Here's how the part is built. I have some questions about the finished solid (model axes, mm). Face numbers are marked on the shaded views. Round coordinates to 2 decimals unless told otherwise and drop trailing zeros. Loops run counter-clockwise (first coordinate to the right, second up) from the corner with the lowest first, then second, coordinate; pieces in that order, holes last. Notation, with made-up numbers: M -39.75,49.5 L -5.75,49.5 A22 cw -5.75,73.5 Z; hole C 4,36.5 d4. An arc over 180 degrees is marked long. Answer as a JSON object with one key per item and string values.
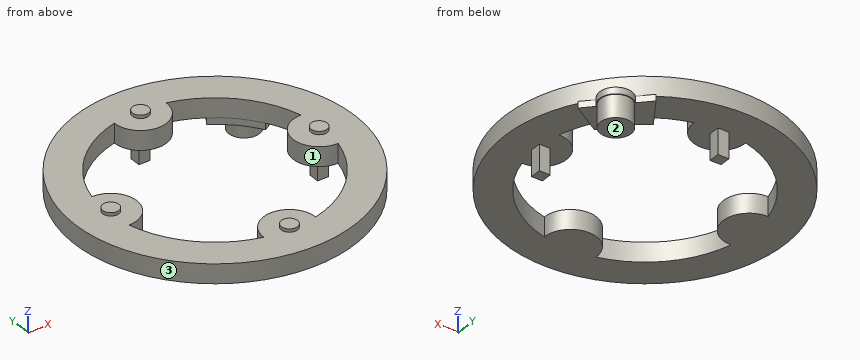
from build123d import *

# Parameters (mm, degrees)
SKETCH1_R           = 110.363
BOSS_EXTRUDE1_DEPTH = 15.24
SKETCH2_R           = 6.35
BOSS_EXTRUDE2_DEPTH = 2.54
SKETCH3_W           = 8.636
SKETCH3_H           = 8.636
BOSS_EXTRUDE3_DEPTH = 20.32
SKETCH4_W           = 8.7122
SKETCH4_H           = 8.636
BOSS_EXTRUDE4_DEPTH = 20.32
BOSS_EXTRUDE5_START = 5.08
BOSS_EXTRUDE5_DEPTH = 5.08
BOSS_EXTRUDE6_DEPTH = 5.08
SKETCH7_R           = 12.070643518
BOSS_EXTRUDE7_DEPTH = 17.78
SCALE2_SCALE        = 1.5


with BuildPart() as part:
    # Sketch1 → Boss-Extrude1 (new body)
    with BuildSketch(Plane.XY):
        Circle(SKETCH1_R)
        with BuildLine():
            ThreePointArc((-20.468919413, 82.460503922), (-60.07791345, 60.07791345), (-82.460503922, 20.468919413))
            ThreePointArc((-82.460503922, 20.468919413), (-61.684540449, 0), (-82.460503922, -20.468919413))
            ThreePointArc((-82.460503922, -20.468919413), (-60.07791345, -60.07791345), (-20.468919413, -82.460503922))
            ThreePointArc((-20.468919413, -82.460503922), (0, -61.684540449), (20.468919413, -82.460503922))
            ThreePointArc((20.468919413, -82.460503922), (60.07791345, -60.07791345), (82.460503922, -20.468919413))
            ThreePointArc((82.460503922, -20.468919413), (61.684540449, 0), (82.460503922, 20.468919413))
            ThreePointArc((82.460503922, 20.468919413), (60.07791345, 60.07791345), (20.468919413, 82.460503922))
            ThreePointArc((20.468919413, 82.460503922), (0, 61.684540449), (-20.468919413, 82.460503922))
        make_face(mode=Mode.SUBTRACT)
    extrude(amount=BOSS_EXTRUDE1_DEPTH)

    # Sketch2 → Boss-Extrude2 (add)
    with BuildSketch(Plane.XY.offset(15.24)):
        with Locations((0, 82.155728736)):
            Circle(SKETCH2_R)
        with Locations((82.155728736, 0)):
            Circle(SKETCH2_R)
        with Locations((0, -82.155728736)):
            Circle(SKETCH2_R)
        with Locations((-82.155728736, 0)):
            Circle(SKETCH2_R)
    extrude(amount=BOSS_EXTRUDE2_DEPTH)

    # Sketch3 → Boss-Extrude3 (add)
    with BuildSketch(Plane(origin=(0, 0, 0), x_dir=(-1, 0, 0), z_dir=(0, 0, -1))):
        with Locations((-82.155728736, 0)):
            Rectangle(SKETCH3_W, SKETCH3_H)
    extrude(amount=BOSS_EXTRUDE3_DEPTH)

    # Sketch4 → Boss-Extrude4 (add)
    with BuildSketch(Plane(origin=(0, 0, 0), x_dir=(-1, 0, 0), z_dir=(0, 0, -1))):
        with Locations((0, 82.155728736)):
            Rectangle(SKETCH4_W, SKETCH4_H)
    extrude(amount=BOSS_EXTRUDE4_DEPTH)

    # Sketch5 → Boss-Extrude5 (add)
    with BuildSketch(Plane(origin=(0, 0, 0), x_dir=(-1, 0, 0), z_dir=(0, 0, -1)).offset(BOSS_EXTRUDE5_START)):
        with BuildLine():
            Line((-72.079043308, 44.981361527), (-95.54887759, 59.627853106))
            Line((-95.54887759, 59.627853106), (-59.627853106, 95.54887759))
            Line((-59.627853106, 95.54887759), (-44.981361527, 72.079043308))
            ThreePointArc((-44.981361527, 72.079043308), (-60.07791345, 60.07791345), (-72.079043308, 44.981361527))
        make_face()
    extrude(amount=-BOSS_EXTRUDE5_DEPTH)

    # Sketch6 → Boss-Extrude6 (add)
    with BuildSketch(Plane(origin=(0, 0, -5.08), x_dir=(-1, 0, 0), z_dir=(0, 0, -1))):
        with BuildLine():
            Line((-87.073217452, 68.103513244), (-69.11270521, 86.064025486))
            ThreePointArc((-69.11270521, 86.064025486), (-87.073217452, 86.064025486), (-87.073217452, 68.103513244))
        make_face()
    extrude(amount=-BOSS_EXTRUDE6_DEPTH)

    # Sketch7 → Boss-Extrude7 (add)
    with BuildSketch(Plane(origin=(0, 0, -5.08), x_dir=(-1, 0, 0), z_dir=(0, 0, -1))):
        with Locations(Location((-78.092961331, 77.083769365, 0), (0, 0, 180))):
            Circle(SKETCH7_R)
    extrude(amount=BOSS_EXTRUDE7_DEPTH)


with BuildPart() as part_1:
    # Scale2: scaled about (4.191580163, 4.163736675, 6.658412252)
    add(part.part.scale(SCALE2_SCALE).moved(Location((-2.095790082, -2.081868337, -3.329206126))))


solid = part_1.part
Item 1: I'm going to push flat-ended pins straight in: pin 1 Ø10.5 at (x, z) = (-2.5, -18) entering from -Y; pin 2 Ø4 at (y, z) = (120, -13) entering from -X; pin 3 Ø14.5 at (x, z) = (-4.5, -25) entering from +Y. Where does each tip first touch, or does it pass through?
Resolved:
{"pin 1": "y = 114.67", "pin 2": "x = -8.63", "pin 3": "y = 127.63"}
Item 2: Please list where these lines run through material, in increasing order: probe 1 along X at (y, z) = (-6, -32); probe 2 along X at (y, z) = (-13.5, -3); probe 3 along Z at (x, y) = (-147.5, 6). Write a range as from..to.
Resolved:
{"probe 1": "114.66..127.61", "probe 2": "-167.25..-96.82, 92.63..163.05", "probe 3": "-3.33..19.53"}
Item 3: I want a section at C-C, the plane z = -27.5. Please give me the cut outline in (x, y), then the cut area to 3 significant figures.
Resolved:
{"outline": "M -8.63,114.67 L 4.44,114.67 L 4.44,127.63 L -8.63,127.63 Z; C 115.04,113.54 d36.21; M 114.66,-8.56 L 127.61,-8.56 L 127.61,4.4 L 114.66,4.4 Z", "area": "1,370 mm²"}
Item 4: If we mould it in two halves opening along X, with no side actions, what happens to the marked faces 1, 2 and 3? For each: pulls with the +X half, pulls with the -X half, needs draft (parallel to the pull), parting line crosses it, or undercut.
Resolved:
{"face 1": "undercut", "face 2": "needs draft", "face 3": "parting line crosses it"}
Item 5: I want a section at B-B, the plane x = -62.5. Please give me the cut outline in (y, z).
Resolved:
{"outline": "M -156.21,-3.33 L -114.3,-3.33 L -114.3,19.53 L -156.21,19.53 Z; M 110.14,-3.33 L 152.05,-3.33 L 152.05,19.53 L 110.14,19.53 Z"}
Item 6: I want a section at D-D, the plane z = 3.5. Please give me the cut outline in (x, y).
Resolved:
{"outline": "C -2.1,-2.08 d331.09; hole M -125.79,-32.79 A127.44 ccw -32.8,-125.77 A30.71 cw long 28.61,-125.77 A127.44 ccw 121.59,-32.79 A30.71 cw long 121.59,28.62 A127.44 ccw 28.61,121.61 A30.71 cw long -32.8,121.61 A127.44 ccw -125.79,28.62 A30.71 cw long Z"}
Item 7: I want a section at A-A, the plane y = -80.5. Please give me the cut outline in (x, z).
Resolved:
{"outline": "M -147.89,-3.33 L -102.56,-3.33 L -102.56,19.53 L -147.89,19.53 Z; M 98.37,-3.33 L 143.7,-3.33 L 143.7,19.53 L 98.37,19.53 Z"}
